For this review, use the dimensioned drawing (mm, ordinates from the lowest corner) and the shaded views. A direction names the side the tool comes from. Round coordinates to 2 decimals unless told otherwise and drop trailing zeros. Write each loop counter-clockwise with the first axis right and the second up, starting at its lowest first coordinate (ties: lowest second). Pieces come first, ordered by that corner, then holes. Notation, with made-up numbers: M 13,-9.5 L 53,-9.5 A19 cw 53,23.5 Z; hole C 11,26 d2. An arc over 180 degrees is marked long. Use one line per item in the form item = value. Start each with the question number.
Item 1: Add section C-C (x = 39). State the section outline as (y, z) points, and give its area (3 significant figures).
Item 2: Add section B-B (z = 38.5). State the section outline as (x, y) points, and give its area (3 significant figures).
Item 3: For P1, Ø3, axis at y = 26.5, z = 30, coming from the -X side; P2, Ø22.5, axis at x = 8, z = 17.5, coming from the +Y side; P3, Ø9.5, axis at x = 43.5, z = 38, coming from the -Y side, all flat-tipped, find the tip position at first contact; note any pin that passes through.
Item 4: Add section A-A (y = 34.5). State the section outline as (x, z) points, and give its area (3 significant figures).
Item 5: Add section D-D (y = 11). State the section outline as (x, z) points, and give its area (3 significant figures).
Item 6: For line 1 (Z direction, x = 5.5, y = 26.5); line 2 (Y direction, x = 18, z = 15); line 3 (Z direction, x = 12, y = 33.5), list the stretches that pass through material, from the lowest coordinate up. Write a range as [from, to].
Item 7: For the marked faces 1, 2 and 3, list the 3-axis set-ups (+Z, -Z, +X, -X, +Y, -Y) from which the entire face can be reached by the end or side of a thin tool; tool diameter is ignored.
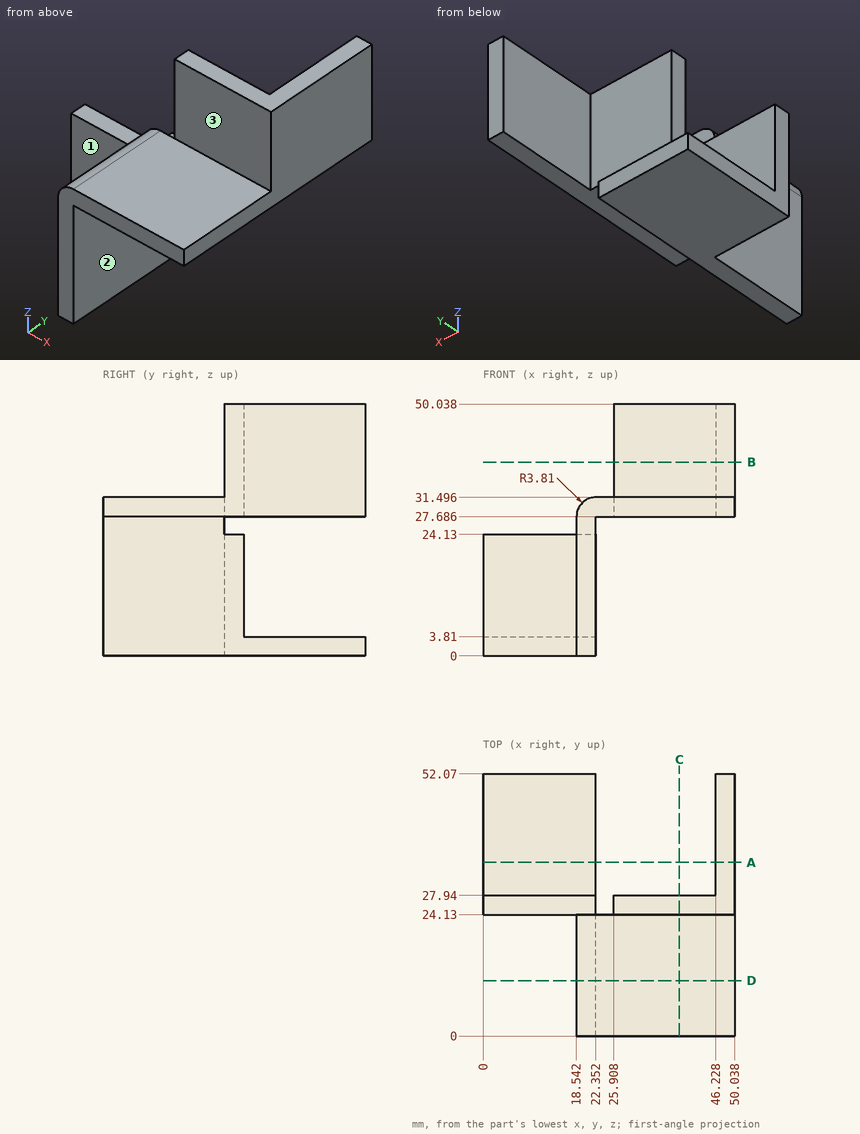
Calculated:
q1.outline = M 0,27.69 L 27.94,27.69 L 27.94,50.04 L 24.13,50.04 L 24.13,31.5 L 0,31.5 Z
q1.area = 177 mm^2
q2.outline = M 25.91,24.13 L 50.04,24.13 L 50.04,52.07 L 46.23,52.07 L 46.23,27.94 L 25.91,27.94 Z
q2.area = 184 mm^2
q3.P1 = 25.91
q3.P2 = 27.94
q3.P3 = 24.13
q4.outline = M 0,0 L 22.35,0 L 22.35,3.81 L 0,3.81 Z; M 46.23,27.69 L 50.04,27.69 L 50.04,50.04 L 46.23,50.04 Z
q4.area = 170 mm^2
q5.outline = M 18.54,0 L 22.35,0 L 22.35,27.69 L 50.04,27.69 L 50.04,31.5 L 22.35,31.5 A3.81 ccw 18.54,27.69 Z
q5.area = 222 mm^2
q6.line_1 = [0, 24.13]
q6.line_2 = [24.13, 27.94]
q6.line_3 = [0, 3.81]
q7.face_1 = +Z, -Z, -X, -Y
q7.face_2 = -Z, +X, +Y, -Y
q7.face_3 = +Z, +X, -X, -Y
